```python
from build123d import *

# Parameters (mm, degrees)
F0_W     = 406.4
F0_H     = 228.6
F0_W_2   = 396.875
F0_H_2   = 219.075
F0_R     = 3.175
F0_R_2   = 13.49375
F0_R_3   = 19.685
F1_DEPTH = 4.7752


# Not quite as in the source:
# - a fillet or chamfer that OpenCascade refuses, or shapes differently, is made with other operations: its cross-section is extruded or revolved along the edge and cut away or added


with BuildPart() as f1:
    # F0 (on Top) → F1 (new body)
    with BuildSketch(Plane.XY):
        with Locations((-26.3652, 4.7498)):
            Rectangle(F0_W, F0_H)
        with Locations((-26.3525, 4.7625)):
            Rectangle(F0_W_2, F0_H_2, mode=Mode.SUBTRACT)
        with Locations((-26.3525, 4.7625)):
            Rectangle(F0_W_2, F0_H_2)
        with Locations((-215.265, -95.25)):
            Circle(F0_R, mode=Mode.SUBTRACT)
        with Locations((-40.64, -25.4)):
            Circle(F0_R_2, mode=Mode.SUBTRACT)
        with Locations((-72.39, 0)):
            Circle(F0_R_2, mode=Mode.SUBTRACT)
        with Locations((162.56, -95.25)):
            Circle(F0_R, mode=Mode.SUBTRACT)
        with Locations((22.86, -25.4)):
            Circle(F0_R_2, mode=Mode.SUBTRACT)
        with Locations((-8.89, 0)):
            Circle(F0_R_2, mode=Mode.SUBTRACT)
        with Locations((54.61, 0)):
            Circle(F0_R_2, mode=Mode.SUBTRACT)
        with Locations((86.36, -25.4)):
            Circle(F0_R_2, mode=Mode.SUBTRACT)
        with Locations((149.86, -25.4)):
            Circle(F0_R_2, mode=Mode.SUBTRACT)
        with Locations((118.11, 0)):
            Circle(F0_R_2, mode=Mode.SUBTRACT)
        with Locations((-183.515, 47.625)):
            Circle(F0_R_3, mode=Mode.SUBTRACT)
        with Locations((-215.265, 104.775)):
            Circle(F0_R, mode=Mode.SUBTRACT)
        with Locations((162.56, 104.775)):
            Circle(F0_R, mode=Mode.SUBTRACT)
    extrude(amount=F1_DEPTH)

    # F2: chamfer of 5.08 on 4 edges, made by hand

    # F2_s1 → F2_t2 (revolve, cut)
    with BuildSketch(Plane.XZ.offset(95.25)):
        Polygon((-212.09, -0.3048), (-207.01, 4.7752), (-212.09, 4.7752), align=None)
    revolve(axis=Axis((-215.265, -95.25, 4.7752), (0, 0, 1)), mode=Mode.SUBTRACT)

    # F2_s3 → F2_t4 (revolve, cut)
    with BuildSketch(Plane.XZ.offset(-104.775)):
        Polygon((-212.09, -0.3048), (-207.01, 4.7752), (-212.09, 4.7752), align=None)
    revolve(axis=Axis((-215.265, 104.775, 4.7752), (0, 0, 1)), mode=Mode.SUBTRACT)

    # F2_s5 → F2_t6 (revolve, cut)
    with BuildSketch(Plane.XZ.offset(-104.775)):
        Polygon((165.735, -0.3048), (170.815, 4.7752), (165.735, 4.7752), align=None)
    revolve(axis=Axis((162.56, 104.775, 4.7752), (0, 0, 1)), mode=Mode.SUBTRACT)

    # F2_s7 → F2_t8 (revolve, cut)
    with BuildSketch(Plane.XZ.offset(95.25)):
        Polygon((165.735, -0.3048), (170.815, 4.7752), (165.735, 4.7752), align=None)
    revolve(axis=Axis((162.56, -95.25, 4.7752), (0, 0, 1)), mode=Mode.SUBTRACT)


solid = f1.part
```
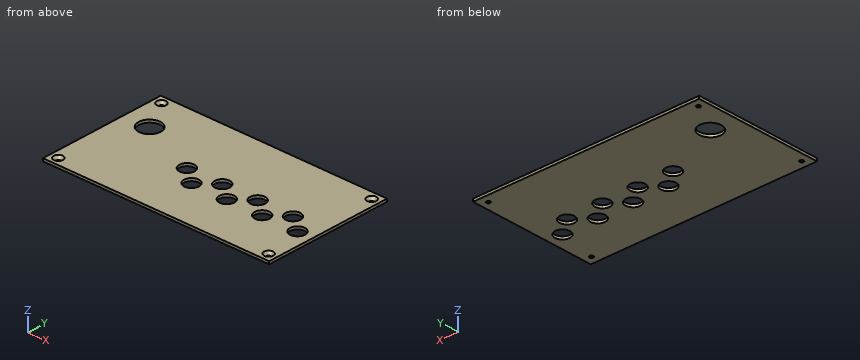
Geometry: final body of the model. Coordinates: model frame, mm. Coordinates: 2 decimals unless noted, no trailing zeros. Order: outer loops, then holes, each group sorted by start corner. A loop starts at its lowest first (then second) coordinate and runs counter-clockwise, first axis right, second up. Notation, with made-up numbers: (41.5, 22) - (88.5, 22) arc R17 cw to (88.5, 27) - close; hole circle Ø2 at (40.5, -15). An arc over 180 degrees is marked (long way). Return JSON: item names as keys, results as strings. Group by question number.
1. Material intervals for line 1 along X through (y, z) = (1.5, 1.6); line 2 along Y through (x, z) = (118.11, 2.75); line 3 along X through (y, z) = (106.5, 3.7), sorted ascending. Write a range as [from, to].
2. Cut plane B-B (y = -25.4). Output: boundary loops of the cut face in (x, z).
3. Cut plane C-C (z = 0.75). Count the separate pieces of the cut face and the enclosed holes in it, plus the area to 3 significant figures.
4. Cut plane A-A (x = 54.61). Output: boundary loops of the cut face in (y, z).
5. Cut plane D-D (y = 57.5). Output: boundary loops of the cut face in (x, z), plus the area to 3 significant figures.
Resolved:
{
 "1": {"line 1": "x = [-229.57, -85.8], [-58.98, -22.3], [4.52, 41.2], [68.02, 104.7], [131.52, 176.83]", "line 2": "y = [-109.55, -13.49], [13.49, 119.05]", "line 3": "x = [-229.57, -222.23], [-208.3, 155.59], [169.53, 176.83]"},
 "2": {"outline": "(-229.57, 0) - (-54.13, 0) - (-54.13, 4.78) - (-229.57, 4.78) - close; (-27.15, 0) - (9.37, 0) - (9.37, 4.78) - (-27.15, 4.78) - close; (36.35, 0) - (72.87, 0) - (72.87, 4.78) - (36.35, 4.78) - close; (99.85, 0) - (136.37, 0) - (136.37, 4.78) - (99.85, 4.78) - close; (163.35, 0) - (176.83, 0) - (176.83, 4.78) - (163.35, 4.78) - close"},
 "3": {"separate pieces": "1", "enclosed holes": "13", "area": "86,900 mm²"},
 "4": {"outline": "(-109.55, 0) - (-13.49, 0) - (-13.49, 4.78) - (-109.55, 4.78) - close; (13.49, 0) - (119.05, 0) - (119.05, 4.78) - (13.49, 4.78) - close"},
 "5": {"outline": "(-229.57, 0) - (-200.54, 0) - (-200.54, 4.78) - (-229.57, 4.78) - close; (-166.49, 0) - (176.83, 0) - (176.83, 4.78) - (-166.49, 4.78) - close", "area": "1,780 mm²"}
}
